from build123d import *

# Parameters (mm, degrees)
SCHIZZO1_R                   = 6
ESTRUSIONE_ESTRUSIONE1_DEPTH = 25
SMUSSO1_SIZE                 = 1
SCHIZZO6_R                   = 9
ESTRUSIONE_ESTRUSIONE3_DEPTH = 12
TAGLIO_ESTRUSIONE3_DEPTH     = 8
SCHIZZO8_R                   = 5.773502692
TAGLIO_ESTRUSIONE4_DEPTH     = 1
TAGLIO_ESTRUSIONE4_TAPER     = 43
RACCORDO4_R                  = 0.5
SCHIZZO9_R                   = 12
SCHIZZO9_R_2                 = 9
ESTRUSIONE_ESTRUSIONE4_DEPTH = 2
RACCORDO5_R                  = 0.2


with BuildPart() as part:
    # Schizzo1 → Estrusione-Estrusione1 (new body)
    with BuildSketch(Plane.XY):
        Circle(SCHIZZO1_R)
    extrude(amount=ESTRUSIONE_ESTRUSIONE1_DEPTH)

    # Smusso1
    smusso1_edges = [part.edges().sort_by_distance(p)[0] for p in [
        (-6, 0, 0),
    ]]
    chamfer(smusso1_edges, length=SMUSSO1_SIZE)

    # Schizzo6 → Estrusione-Estrusione3 (add)
    with BuildSketch(Plane.XY.offset(25)):
        Circle(SCHIZZO6_R)
    extrude(amount=ESTRUSIONE_ESTRUSIONE3_DEPTH)

    # Schizzo7 → Taglio-Estrusione3 (cut)
    with BuildSketch(Plane.XY.offset(37)):
        Polygon((2.886751346, 5), (-2.886751346, 5), (-5.773502692, 0), (-2.886751346, -5), (2.886751346, -5), (5.773502692, 0), align=None)
    extrude(amount=-TAGLIO_ESTRUSIONE3_DEPTH, mode=Mode.SUBTRACT)

    # Schizzo8 → Taglio-Estrusione4 (cut)
    with BuildSketch(Plane.XY.offset(37)):
        Circle(SCHIZZO8_R)
    extrude(amount=-TAGLIO_ESTRUSIONE4_DEPTH, taper=TAGLIO_ESTRUSIONE4_TAPER, mode=Mode.SUBTRACT)

    # Raccordo4
    raccordo4_edges = [part.edges().sort_by_distance(p)[0] for p in [
        (-9, 0, 37),
    ]]
    fillet(raccordo4_edges, radius=RACCORDO4_R)

    # Schizzo9 → Estrusione-Estrusione4 (add)
    with BuildSketch(Plane(origin=(0, 0, 25), x_dir=(-1, 0, 0), z_dir=(0, 0, -1))):
        Circle(SCHIZZO9_R)
        Circle(SCHIZZO9_R_2, mode=Mode.SUBTRACT)
    extrude(amount=-ESTRUSIONE_ESTRUSIONE4_DEPTH)

    # Raccordo5
    raccordo5_edges = [part.edges().sort_by_distance(p)[0] for p in [
        (-9, 0, 27),
        (12, 0, 27),
        (12, 0, 25),
    ]]
    fillet(raccordo5_edges, radius=RACCORDO5_R)


solid = part.part
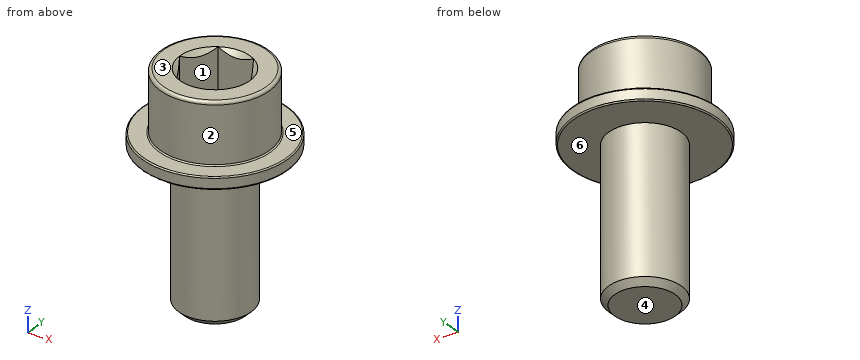
Check sheet for the modelled part. Datum: model origin and axes. Units: mm. Face numbers are marked on the shaded views. A direction names the side the tool comes from. Round coordinates to 2 decimals unless told otherwise and drop trailing zeros. Order: outer loops, then holes, each group sorted by start corner. A loop starts at its lowest first (then second) coordinate and runs counter-clockwise, first axis right, second up.
(1) Access from +Z, -Z, +X, -X, +Y, -Y to the whole of each face (thin tool, end or side, straight path). Record for the marked faces 4, 5 and 6.
(2) Cross-section at A-A, the plane z = 31. Enter the section's corners in (x, y).
(3) Go/stop test with flat-tipped pins: P1, Ø12, axis at y = 7, z = 13, coming from the +X side; P2, Ø8, axis at y = 4.5, z = 26.5, coming from the +X side; P3, Ø5, axis at x = 3, y = 7, coming from the -Z side. Record where each tip stops, or that it passes through.
(4) Cross-section at D-D, the plane z = 26. Enter the section's corners in (x, y), and give its area (3 significant figures).
(5) Draft check along X on the marked faces 1, 2 and 3. Enter one of: pulls with the +X half, pulls with the -X half, needs draft (parallel to the pull), parting line crosses it, or undercut.
(6) Cross-section at C-C, the plane z = 2.5. Enter the section's corners in (x, y), and give its area (3 significant figures).
(7) Scan lines: probe 1 along Y at (x, z) = (0, 32); probe 2 along Z at (x, y) = (7, 6.25); probe 3 along Z at (x, y) = (-2, 5.75). Record each from-to range of solid material in increasing order.
(8) Cross-section at B-B, the plane x = 0. Enter the section's corners in (y, z).
Check sheet entries:
1. face 4: -Z, +X, -X, +Y, -Y
1. face 5: +Z
1. face 6: -Z
2. outline: circle Ø18 at (0, 0); hole (-5.77, 0) - (-2.89, -5) - (2.89, -5) - (5.77, 0) - (2.89, 5) - (-2.89, 5) - close
3. P1: stops at x = 5.92
3. P2: stops at x = 11.99
3. P3: stops at z = 0.12
4. outline: circle Ø24 at (0, 0)
4. area: 452 mm2
5. face 1: undercut
5. face 2: parting line crosses it
5. face 3: needs draft
6. outline: circle Ø12 at (0, 0)
6. area: 113 mm2
7. probe 1: y = -9 to -5, 5 to 9
7. probe 2: z = 25 to 27
7. probe 3: z = 25 to 37
8. outline: (-12, 25.2) arc R0.2 ccw to (-11.8, 25) - (-6, 25) - (-6, 1) - (-5, 0) - (5, 0) - (6, 1) - (6, 25) - (11.8, 25) arc R0.2 ccw to (12, 25.2) - (12, 26.8) arc R0.2 ccw to (11.8, 27) - (9.2, 27) arc R0.2 cw to (9, 27.2) - (9, 36.5) arc R0.5 ccw to (8.5, 37) - (5.77, 37) - (5, 36.17) - (5, 29) - (-5, 29) - (-5, 36.17) - (-5.77, 37) - (-8.5, 37) arc R0.5 ccw to (-9, 36.5) - (-9, 27.2) arc R0.2 cw to (-9.2, 27) - (-11.8, 27) arc R0.2 ccw to (-12, 26.8) - close
